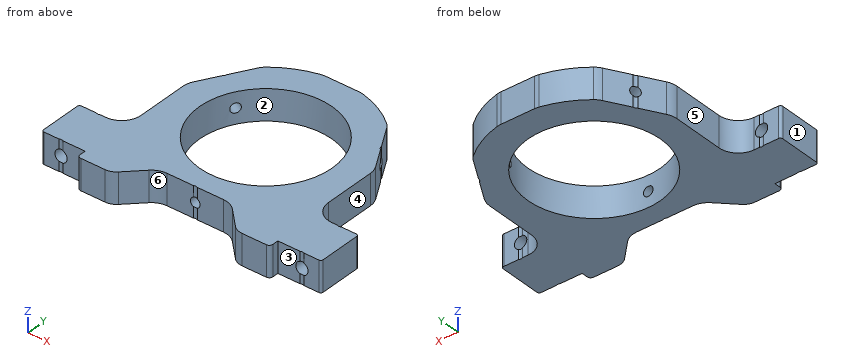
from build123d import *

# Parameters (mm, degrees)
SKETCH1_R           = 27.500000001
BOSS_EXTRUDE1_DEPTH = 12.7
SKETCH2_R           = 2.55
CUT_EXTRUDE1_DEPTH  = 406.309199291
SKETCH4_R           = 2
CUT_EXTRUDE2_DEPTH  = 15
SKETCH5_R           = 2
CUT_EXTRUDE3_DEPTH  = 15
SKETCH3_R           = 2
CUT_EXTRUDE4_DEPTH  = 15


with BuildPart() as part:
    # Sketch1 → Boss-Extrude1 (new body)
    with BuildSketch(Plane.XY):
        with BuildLine():
            Line((284.236473266, 94.417355971), (284.236473266, 77.41735597))
            ThreePointArc((284.236473266, 77.41735597), (284.529366484, 76.71024919), (285.236473265, 76.417355971))
            Line((285.236473265, 76.417355971), (291.410292076, 76.417355971))
            ThreePointArc((291.410292076, 76.417355971), (292.236473265, 76.642955971), (293.062654455, 76.417355971))
            Line((293.062654455, 76.417355971), (302.236473265, 76.417355971))
            Line((302.236473265, 76.417355971), (302.236473265, 73.91735597))
            ThreePointArc((302.236473265, 73.91735597), (302.675813094, 72.856695799), (303.736473265, 72.41735597))
            Line((303.736473265, 72.41735597), (313.751191892, 72.41735597))
            ThreePointArc((313.751191892, 72.41735597), (316.047292486, 72.874078775), (317.993832578, 74.174715283))
            Line((317.993832578, 74.174715283), (324.893327515, 81.074210219))
            ThreePointArc((324.893327515, 81.074210219), (327.488714305, 82.80839223), (330.550181764, 83.417355969))
            Line((330.550181764, 83.417355969), (341.410292075, 83.417355969))
            ThreePointArc((341.410292075, 83.417355969), (342.236473267, 83.642955969), (343.062654458, 83.417355968))
            Line((343.062654458, 83.417355968), (353.922764767, 83.417355968))
            ThreePointArc((353.922764767, 83.417355968), (356.984232225, 82.808392228), (359.579619016, 81.074210218))
            Line((359.579619016, 81.074210218), (366.479113952, 74.174715282))
            ThreePointArc((366.479113952, 74.174715282), (368.425654045, 72.874078773), (370.72175464, 72.417355968))
            Line((370.72175464, 72.417355968), (380.736473265, 72.417355968))
            ThreePointArc((380.736473265, 72.417355968), (381.797133436, 72.856695796), (382.236473264, 73.917355967))
            Line((382.236473264, 73.917355967), (382.236473264, 76.417355972))
            Line((382.236473264, 76.417355972), (391.410292073, 76.417355972))
            ThreePointArc((391.410292073, 76.417355972), (392.236473265, 76.642955972), (393.062654456, 76.417355971))
            Line((393.062654456, 76.417355971), (399.236473264, 76.417355971))
            ThreePointArc((399.236473264, 76.417355971), (399.943580044, 76.71024919), (400.236473263, 77.41735597))
            Line((400.236473263, 77.41735597), (400.236473263, 94.417355971))
            ThreePointArc((400.236473263, 94.417355971), (399.943580044, 95.124462751), (399.236473264, 95.41735597))
            Line((399.236473264, 95.41735597), (393.062654456, 95.41735597))
            ThreePointArc((393.062654456, 95.41735597), (392.236473265, 95.191755969), (391.410292073, 95.417355969))
            Line((391.410292073, 95.417355969), (389.110963045, 95.417355969))
            ThreePointArc((389.110963045, 95.417355969), (383.454108795, 97.760501719), (381.110963044, 103.417355969))
            Line((381.110963044, 103.417355969), (381.110963044, 124.734871013))
            ThreePointArc((381.110963044, 124.734871013), (380.838369654, 126.805423374), (380.039166274, 128.734871013))
            Line((380.039166274, 128.734871013), (375.125516501, 137.245562071))
            ThreePointArc((375.125516501, 137.245562071), (374.517050575, 137.848255971), (374.299335311, 138.676549871))
            Line((374.299335311, 138.676549871), (369.016145298, 147.8273034))
            ThreePointArc((369.016145298, 147.8273034), (368.165927768, 149.029042515), (367.109909002, 150.054650194))
            ThreePointArc((367.109909002, 150.054650194), (359.459956736, 154.89532039), (350.910948847, 157.873293146))
            ThreePointArc((350.910948847, 157.873293146), (350.040616408, 158.018692254), (349.159565162, 158.06735597))
            Line((349.159565162, 158.06735597), (335.313381368, 158.06735597))
            ThreePointArc((335.313381368, 158.06735597), (334.432330122, 158.018692254), (333.561997683, 157.873293146))
            ThreePointArc((333.561997683, 157.873293146), (325.012989794, 154.89532039), (317.363037528, 150.054650194))
            ThreePointArc((317.363037528, 150.054650194), (316.307018762, 149.029042515), (315.456801232, 147.8273034))
            Line((315.456801232, 147.8273034), (310.173611219, 138.676549871))
            ThreePointArc((310.173611219, 138.676549871), (309.955895955, 137.848255971), (309.34743003, 137.245562072))
            Line((309.34743003, 137.245562072), (304.433780256, 128.734871013))
            ThreePointArc((304.433780256, 128.734871013), (303.634576876, 126.805423374), (303.361983486, 124.734871013))
            Line((303.361983486, 124.734871013), (303.361983486, 103.417355969))
            ThreePointArc((303.361983486, 103.417355969), (301.018837735, 97.76050172), (295.361983486, 95.41735597))
            Line((295.361983486, 95.41735597), (293.062654455, 95.41735597))
            ThreePointArc((293.062654455, 95.41735597), (292.236473265, 95.19175597), (291.410292076, 95.41735597))
            Line((291.410292076, 95.41735597), (285.236473265, 95.41735597))
            ThreePointArc((285.236473265, 95.41735597), (284.529366484, 95.124462751), (284.236473266, 94.417355971))
        make_face()
        with Locations((342.236473265, 119.21105597)):
            Circle(SKETCH1_R, mode=Mode.SUBTRACT)
    extrude(amount=BOSS_EXTRUDE1_DEPTH)

    # Sketch2 → Cut-Extrude1 (cut, through all)
    with BuildSketch(Plane(origin=(0, 95.41735597, 0), x_dir=(1, 0, 0), z_dir=(0, 1, 0))):
        with Locations(Location((292.236473265, -6.35, 0), (0, 0, 288.904554562))):
            Circle(SKETCH2_R)
        with Locations(Location((392.236473265, -6.35, 0), (0, 0, 288.904554598))):
            Circle(SKETCH2_R)
    extrude(amount=-CUT_EXTRUDE1_DEPTH, mode=Mode.SUBTRACT)

    # Sketch4 → Cut-Extrude2 (cut)
    with BuildSketch(Plane(origin=(172.581500867, -99.639975983, 0), x_dir=(0, 0, 1), z_dir=(-0.8660254037844396, 0.49999999999999856, 0))):
        with Locations(Location((6.35, 274.358039516, 0), (0, 0, 270))):
            Circle(SKETCH4_R)
    extrude(amount=-CUT_EXTRUDE2_DEPTH, mode=Mode.SUBTRACT)

    # Sketch5 → Cut-Extrude3 (cut)
    with BuildSketch(Plane(origin=(340.773209032, 196.745503967, 0), x_dir=(0, 0, -1), z_dir=(0.8660254037844377, 0.5000000000000019, 0))):
        with Locations(Location((-6.35, -67.87843375, 0), (0, 0, 90))):
            Circle(SKETCH5_R)
    extrude(amount=-CUT_EXTRUDE3_DEPTH, mode=Mode.SUBTRACT)

    # Sketch3 → Cut-Extrude4 (cut)
    with BuildSketch(Plane.XZ.offset(-83.417355968)):
        with Locations(Location((342.236473266, 6.35, 0), (0, 0, 270))):
            Circle(SKETCH3_R)
    extrude(amount=-CUT_EXTRUDE4_DEPTH, mode=Mode.SUBTRACT)


solid = part.part
Model file for the job. Use its own axes, mm. Face numbers are marked on the shaded views. A direction names the side the tool comes from. Give positions to 0.01 mm unless a question says otherwise; leave off trailing zeros. Loops run counter-clockwise (first coordinate to the right, second up) from the corner with the lowest first, then second, coordinate; pieces in that order, holes last.
1) Saw through at A-A (y = 130). Write the cut outline in (x, z), plus the area to 3 significant figures.
2) Flat gauge pins, fed straight in: pin 1 Ø1.3 at (y, z) = (75.5, 6.5) entering from +X; pin 2 Ø3.5 at (x, z) = (347, 7) entering from -Y; pin 3 Ø2.5 at (x, z) = (389.5, 7) entering from +Y; pin 4 Ø10 at (x, y) = (325.5, 107) entering from -Z. Where does each tip first touch, or does it go through?
3) Pull direction X, two halves, no side cores. Call the marked faces 1, 2 and 3: +X half, -X half, draft (parallel to the pull), parting line (faces both ways), or undercut.
4) Saw through at B-B (x = 332). Write the cut outline in (y, z), plus the area to 3 significant figures.
5) Saw through at C-C (z = 6.35). Count the separate pieces of the cut face and the enclosed holes in it, plus the area to 3 significant figures.
6) Wall check: line 1 (X direction, y = 89.5, z = 6.35); line 2 (Y direction, x = 366, z = 11.5); line 3 (X direction, y = 88.5, z = 5.75). Give the ranges that are in metal, low to high.
7) Tool access for the marked faces 4, 5 and 6: list every direction of +Z, -Z, +X, -X, +Y, -Y with a clear straight run to the whole face (end or side of a thin tool).
Answer block:
1. outline: (305.16, 0) - (316.94, 0) - (316.94, 12.7) - (305.16, 12.7) - close; (367.53, 0) - (379.31, 0) - (379.31, 12.7) - (367.53, 12.7) - close
1. area: 299 mm2
2. pin 1: stops at x = 382.24
2. pin 2: stops at y = 83.42
2. pin 3: stops at y = 95.46
2. pin 4: passes through
3. face 1: -X half
3. face 2: undercut
3. face 3: draft
4. outline: (83.42, 0) - (93.69, 0) - (93.69, 12.7) - (83.42, 12.7) - close; (144.73, 0) - (157.49, 0) - (157.49, 12.7) - (144.73, 12.7) - close
4. area: 292 mm2
5. separate pieces: 5
5. enclosed holes: 0
5. area: 3,640 mm2
6. line 1: x = 284.24 to 289.69, 294.79 to 340.24, 344.24 to 389.69, 394.79 to 400.24
6. line 2: y = 74.65 to 105.37, 133.05 to 150.92
6. line 3: x = 284.24 to 289.76, 294.71 to 340.33, 344.14 to 389.76, 394.71 to 400.24
7. face 4: +Z, -Z, +X, +Y
7. face 5: +Z, -Z, -X, +Y
7. face 6: +Z, -Z, -Y
